```python
from build123d import *

# Parameters (mm, degrees)
EXTRUDE_1_DEPTH             = 11.5
FILLET_1_R                  = 0.3
FILLET_2_R                  = 2
HOLE_WIZARD_M42_D           = 3.3
HOLE_WIZARD_M42_CSINK_D     = 4.3
HOLE_WIZARD_M42_CSINK_ANGLE = 90


with BuildPart() as part:
    # Эскиз1 → Бобышка-Вытянуть1 (new body, symmetric)
    with BuildSketch(Plane.XY):
        with BuildLine():
            Line((-5, 0), (5, 0))
            Line((5, 0), (5, -0.8))
            Line((5, -0.8), (8, -0.8))
            Line((8, -0.8), (8, -1.6))
            ThreePointArc((8, -1.6), (5.309398779, -5.576969864), (1.5, -8.5))
            Line((1.5, -8.5), (-1.5, -8.5))
            ThreePointArc((-1.5, -8.5), (-5.309398779, -5.576969864), (-8, -1.6))
            Line((-8, -1.6), (-8, -0.8))
            Line((-8, -0.8), (-5, -0.8))
            Line((-5, -0.8), (-5, 0))
        make_face()
    extrude(amount=EXTRUDE_1_DEPTH, both=True)

    # Скругление1
    fillet_1_edges = [part.edges().sort_by_distance(p)[0] for p in [
        (8, -0.8, 0),
        (8, -1.6, 0),
        (-8, -1.6, 0),
        (-8, -0.8, 0),
        (-5, 0, 0),
        (5, 0, 0),
    ]]
    fillet(fillet_1_edges, radius=FILLET_1_R)

    # Скругление2
    fillet_2_edges = [part.edges().sort_by_distance(p)[0] for p in [
        (1.5, -8.5, 0),
        (-1.5, -8.5, 0),
    ]]
    fillet(fillet_2_edges, radius=FILLET_2_R)

    # Отверстие обработанное метчиком M42 (through all)
    with Locations(Plane(origin=(0, 0, 0), x_dir=(1, 0, 0), z_dir=(0, 1, 0))):
        with Locations((0, -4.5)):
            CounterSinkHole(HOLE_WIZARD_M42_D / 2, HOLE_WIZARD_M42_CSINK_D / 2, counter_sink_angle=HOLE_WIZARD_M42_CSINK_ANGLE)

    # Эскиз5 → Повернуть1 (revolve)
    with BuildSketch(Plane(origin=(0, 0, 0), x_dir=(0, 0, -1), z_dir=(1, 0, 0))):
        with BuildLine():
            Line((6.5, -4.3), (6.5, -9.3))
            ThreePointArc((6.5, -9.3), (4, -6.8), (6.5, -4.3))
        make_face()
    revolve(axis=Axis((0, -4.3, -6.5), (0, -1, 0)))


solid = part.part
```
The model under review builds one solid part; all positions refer to its coordinate system, in mm. A direction names the side the tool comes from. Give positions to 0.01 mm unless a question says otherwise; leave off trailing zeros. Write each loop counter-clockwise with the first axis right and the second up, starting at its lowest first coordinate (ties: lowest second). Pieces come first, ordered by that corner, then holes. Notation, with made-up numbers: M -39,0.5 L -22,0.5 A16 ccw -22,14.5 Z; hole C 49,49 d8. An arc over 180 degrees is marked long. Write each question's results on one line, items separated by ' | '. Start each with the question number.
1. Mouldability with a two-part tool opening along Z and no side actions: class faces 5 (the flat face through (0, -8.5, -10)), 6 (the flat face through (0, -3, -11.5)), 7 (the cylindrical face through (0.4, -4.6, 6.1)) as released by +Z, released by -Z, zero draft, split by the parting line, or undercut.
2. We need section A-A (z = 8.75). Write out the cut boundary in (x, y).
3. We need section B-B (y = -4.25). Write out the cut boundary in (x, z), and give its area (3 significant figures).
4. We need section C-C (z = 4.5). Write out the cut boundary in (x, y), and give its area (3 significant figures).
5. For probe 1 along Z at (x, y) = (0, -4); probe 2 along X at (y, z) = (-5.5, 4.75); probe 3 along X at (y, z) = (-3, 4.5), list the stretches that pass through material, from the lowest coordinate up. Write a range as [from, to].
6. For faces 1 (the flat face through (0, -8.5, 9)), 2 (the cylindrical face through (-1.509, -8.428, 2.633)), 3 (the cylindrical face through (1.509, -8.428, -9.786)), 4 (the flat face through (6, -0.8, 0)), list the 3-axis set-ups (+Z, -Z, +X, -X, +Y, -Y) from which the entire face can be reached by the end or side of a thin tool; tool diameter is ignored.
7. We need section D-D (x = 6). Write out the cut boundary in (y, z).
8. Insertion check: pin 1 Ø2 at (y, z) = (-5.5, -5) entering from -X; pin 2 Ø4.5 at (x, z) = (0, 4.5) entering from -Y; pin 3 Ø3 at (x, z) = (-6, 2.5) entering from +Y; pin 4 Ø1 at (x, y) = (-6, -7) entering from -Z (1 decimal). Each pin has a flat end and moves straight along its axis. Give the tip position at first contact, or say it passes through.
Results found:
1) face 5: zero draft | face 6: released by -Z | face 7: undercut
2) outline: M -8,-1.53 A0.3 ccw -7.97,-1.66 A15 ccw -1.99,-8.22 A2 ccw -0.98,-8.5 L 0.98,-8.5 A2 ccw 1.99,-8.22 A15 ccw 7.97,-1.66 A0.3 ccw 8,-1.53 L 8,-1.1 A0.3 ccw 7.7,-0.8 L 5,-0.8 L 5,-0.3 A0.3 ccw 4.7,0 L -4.7,0 A0.3 ccw -5,-0.3 L -5,-0.8 L -7.7,-0.8 A0.3 ccw -8,-1.1 Z
3) outline: M -6.42,-11.5 L 6.42,-11.5 L 6.42,11.5 L -6.42,11.5 Z; hole C 0,4.5 d3.3 | area: 287 mm^2
4) outline: M -8,-1.53 A0.3 ccw -7.97,-1.66 A15 ccw -1.99,-8.22 A2 ccw -1.65,-8.38 L -1.65,-0.5 L -2.15,0 L -4.7,0 A0.3 ccw -5,-0.3 L -5,-0.8 L -7.7,-0.8 A0.3 ccw -8,-1.1 Z; M 1.65,-8.38 A2 ccw 1.99,-8.22 A15 ccw 7.97,-1.66 A0.3 ccw 8,-1.53 L 8,-1.1 A0.3 ccw 7.7,-0.8 L 5,-0.8 L 5,-0.3 A0.3 ccw 4.7,0 L 2.15,0 L 1.65,-0.5 Z | area: 67.7 mm^2
5) probe 1: z = [-11.5, 2.85], [6.15, 11.5] | probe 2: x = [-5.38, -1.63], [1.63, 5.38] | probe 3: x = [-7.26, -1.65], [1.65, 7.26]
6) face 1: +Z, +X, -X, -Y | face 2: +Z, -X, -Y | face 3: -Z, +X, -Y | face 4: +Z, -Z, +X, +Y
7) outline: M -4.79,-11.5 L -0.8,-11.5 L -0.8,11.5 L -4.79,11.5 Z
8) pin 1: stops at x = -6.23 | pin 2: stops at y = -8.5 | pin 3: stops at y = 0 | pin 4: passes through
